Source: CAD feature listing. Evaluate the final solid. Frame: model axes, mm. Face numbers are marked on the shaded views. Give positions to 0.01 mm unless a question says otherwise; leave off trailing zeros. Write each loop counter-clockwise with the first axis right and the second up, starting at its lowest first coordinate (ties: lowest second). Pieces come first, ordered by that corner, then holes. Notation, with made-up numbers: (-9.5, 65) -> (33.5, 65) arc R38 cw to (33.5, 104) -> close; hole circle Ø8 at (80.5, 38). An arc over 180 degrees is marked (long way). Use one line per item in the form item = value. Start each with the question number.
(1) Cut plane C-C, the plane y = 0.8. Output: boundary loops of the cut face in (x, z).
(2) First-contact query: P1, Ø1.5, axis at y = 1, z = 6.5, coming from the -X side. Flat tip, straight axial feed; report the tip coordinate or a pass-through.
(3) Cut plane D-D, the plane x = 1.75. Count the separate pieces of the cut face and the enclosed holes in it, and give its area (3 significant figures).
(4) Cut plane B-B, the plane x = 2.5. Output: boundary loops of the cut face in (y, z).
(5) Draft query along Z for the marked faces 1, 2 and 3. Return one class per face: pulls with the +Z half, pulls with the -Z half, needs draft (parallel to the pull), parting line crosses it, or undercut.
(6) Cut plane A-A, the plane z = 10. Output: boundary loops of the cut face in (x, y).
(7) Material intervals for line 1 along Z through (x, y) = (2.5, 0.7); line 2 along X through (y, z) = (1.6, 10); line 3 along Z through (x, y) = (2, 2.2), sorted ascending. Write a range as from..to.
from build123d import *

# Parameters (mm, degrees)
SKETCH_1_W          = 5
SKETCH_1_H          = 15
EXTRUDE_1_DEPTH     = 2.75
SKETCH_2_R          = 1
CUT_EXTRUDE_1_DEPTH = 3.75
CUT_EXTRUDE_2_DEPTH = 16
CHAMFER_1_SIZE      = 0.2


with BuildPart() as part:
    # 草图1 → 凸台-拉伸1 (new body)
    with BuildSketch(Plane(origin=(0, 0, 0), x_dir=(1, 0, 0), z_dir=(0, 1, 0))):
        with Locations((2.5, -7.5)):
            Rectangle(SKETCH_1_W, SKETCH_1_H)
    extrude(amount=EXTRUDE_1_DEPTH)

    # 草图2 → 切除-拉伸1 (cut, through all)
    with BuildSketch(Plane(origin=(0, 0, 0), x_dir=(-1, 0, 0), z_dir=(0, -1, 0))):
        with Locations((-2.5, -10)):
            Circle(SKETCH_2_R)
        with Locations((-2.5, -5)):
            Circle(SKETCH_2_R)
    extrude(amount=-CUT_EXTRUDE_1_DEPTH, mode=Mode.SUBTRACT)

    # 草图3 → 切除-拉伸2 (cut, through all)
    with BuildSketch(Plane(origin=(0, 0, 0), x_dir=(-1, 0, 0), z_dir=(0, 0, -1))):
        Polygon((0, 1.112237097), (-0.183390928, 1.271215949), (0, 1.430194801), align=None)
        Polygon((-5, 1.112237097), (-4.841021148, 1.271215949), (-5, 1.430194801), align=None)
    extrude(amount=-CUT_EXTRUDE_2_DEPTH, mode=Mode.SUBTRACT)

    # 倒角1
    chamfer_1_edges = [part.edges().sort_by_distance(p)[0] for p in [
        (3.5, 2.75, 10),
        (3.5, 2.75, 5),
    ]]
    chamfer(chamfer_1_edges, length=CHAMFER_1_SIZE)


solid = part.part
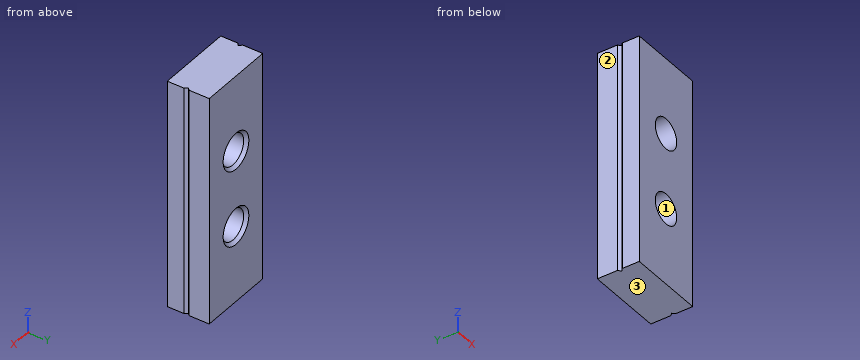
Geometry says:
q1.outline = (0, 0) -> (5, 0) -> (5, 15) -> (0, 15) -> close; hole circle Ø2 at (2.5, 5); hole circle Ø2 at (2.5, 10)
q2.P1 = 0
q3.separate_pieces = 3
q3.enclosed_holes = 0
q3.area = 33.9 mm^2
q4.outline = (0, 0) -> (2.75, 0) -> (2.75, 3.8) -> (2.55, 4) -> (0, 4) -> close; (0, 6) -> (2.55, 6) -> (2.75, 6.2) -> (2.75, 8.8) -> (2.55, 9) -> (0, 9) -> close; (0, 11) -> (2.55, 11) -> (2.75, 11.2) -> (2.75, 15) -> (0, 15) -> close
q5.face_1 = undercut
q5.face_2 = needs draft
q5.face_3 = pulls with the -Z half
q6.outline = (0, 0) -> (1.5, 0) -> (1.5, 2.55) -> (1.3, 2.75) -> (0, 2.75) -> (0, 1.43) -> (0.18, 1.27) -> (0, 1.11) -> close; (3.5, 0) -> (5, 0) -> (5, 1.11) -> (4.84, 1.27) -> (5, 1.43) -> (5, 2.75) -> (3.7, 2.75) -> (3.5, 2.55) -> close
q7.line_1 = 0..4, 6..9, 11..15
q7.line_2 = 0..1.5, 3.5..5
q7.line_3 = 0..4.13, 5.87..9.13, 10.87..15
